Verification items for the finished model (mm, model axes). A direction names the side the tool comes from. Give positions to 0.01 mm unless a question says otherwise; leave off trailing zeros. Use a Markdown table: item, result.
from build123d import *

# Parameters (mm, degrees)
CUT_EXTRUDE_1_DEPTH         = 298.8022876
CUT_EXTRUDE_1_DEPTH_BACK    = 298.8022876
SKETCH_2_W                  = 19
SKETCH_2_H                  = 9.5
SKETCH_3_R                  = 55
EXTRUDE_1_DEPTH             = 1.5125
SKETCH_4_W                  = 19
SKETCH_4_H                  = 9.5
CUT_EXTRUDE_2_DEPTH         = 2
HOLE_WIZARD_M41_D           = 4.5
PATTERN_CIRCULAR_1_COUNT    = 4
HOLE_WIZARD_M42_D           = 4.5
HOLE_WIZARD_M42_CSINK_D     = 4.55
HOLE_WIZARD_M42_CSINK_ANGLE = 90


with BuildPart() as part:
    # Эскиз1 → Повернуть1 (revolve)
    with BuildSketch(Plane(origin=(0, 0, 0), x_dir=(1, 0, 0), z_dir=(0, 1, 0)), mode=Mode.PRIVATE) as revolve_1_sk:
        Polygon((0, 0), (200, 0), (200, -20), (210, -22.05), (210, 10), (0, 10), align=None)
    revolve(revolve_1_sk.sketch.rotate(Axis((0, 0, -10), (0, 0, 1)), 180), axis=Axis((0, 0, -10), (0, 0, 1)))

    # Эскиз2 → Вырез-Вытянуть1 (cut, two sides: drawn at the far end of the back side and taken through both)
    with BuildSketch(Plane.XY.offset(-CUT_EXTRUDE_1_DEPTH_BACK)):
        Rectangle(SKETCH_2_W, SKETCH_2_H)
    extrude(amount=CUT_EXTRUDE_1_DEPTH + CUT_EXTRUDE_1_DEPTH_BACK, mode=Mode.SUBTRACT)

    # Эскиз3 → Бобышка-Вытянуть1 (add)
    with BuildSketch(Plane.XY):
        with Locations(Location((0, 0, 0), (0, 0, 180))):
            Circle(SKETCH_3_R)
    extrude(amount=EXTRUDE_1_DEPTH)

    # Эскиз4 → Вырез-Вытянуть2 (cut)
    with BuildSketch(Plane.XY.offset(1.5125)):
        Rectangle(SKETCH_4_W, SKETCH_4_H)
    extrude(amount=-CUT_EXTRUDE_2_DEPTH, mode=Mode.SUBTRACT)

    # Отверстие с зазором M41 (through all)
    with Locations(Plane(origin=(0, 45, 1.5125), x_dir=(1, 0, 0), z_dir=(0, 0, 1))):
        with Locations((0, 0)):
            hole_wizard_m41 = Hole(HOLE_WIZARD_M41_D / 2)

    # Круговой массив1: Отверстие с зазором M41 ×4 about axis
    pattern_circular_1_axis = Axis((0, 0, 0), (0, 0, 1))
    for i in range(1, PATTERN_CIRCULAR_1_COUNT):
        add(hole_wizard_m41.rotate(pattern_circular_1_axis, i * 360 / PATTERN_CIRCULAR_1_COUNT), mode=Mode.SUBTRACT)

    # Отверстие с зазором M42 (through all)
    with Locations(Plane(origin=(-14.5, 15, -10), x_dir=(-1, 0, 0), z_dir=(0, 0, -1))):
        with Locations((0, 0), (-29, 0), (-29, -30), (0, -30)):
            CounterSinkHole(HOLE_WIZARD_M42_D / 2, HOLE_WIZARD_M42_CSINK_D / 2, counter_sink_angle=HOLE_WIZARD_M42_CSINK_ANGLE)


solid = part.part
(1) Gauge pin test, flat ends, axial feed: P1, Ø8, axis at x = -8, z = 6.5, coming from the +Y side; P2, Ø6, axis at x = 109.5, z = 9.5, coming from the +Y side; P3, Ø10, axis at y = 138.5, z = 14.5, coming from the +X side. Record the tip position at first contact, or that the pin passes through.
Results below:
| item | result |
|---|---|
| P1 | y = 209.96 |
| P2 | y = 180.99 |
| P3 | x = 162.1 |
(2) Set-up check for faces 4 (the flat face through (0, -4.75, -4)), 5 (the flat face through (1, 11, 1.512)): record each of +Z, -Z, +X, -X, +Y, -Y from which the full face is reachable in a straight line by a thin tool's end or side.
Results below:
| item | result |
|---|---|
| face 4 | +Z, -Z |
| face 5 | +Z |
(3) Draft check along X on faces 1 (the cylindrical face through (-200.3, -63.08, 5.8)), 2 (the flat face through (-9.5, 0, -4)), 3 (the flat face through (3, 44, -10)). Enter one of: +X half, -X half, draft (parallel to the pull), parting line (faces both ways), or undercut.
Results below:
| item | result |
|---|---|
| face 1 | parting line |
| face 2 | undercut |
| face 3 | draft |
(4) Material ranges on line 1 (Y direction, x = 0, z = -6); line 2 (X direction, y = -15, z = -6.5); line 3 (Z direction, x = -10, y = -34), recorded low to high.
Results below:
| item | result |
|---|---|
| line 1 | -210 to -47.25, -42.75 to -4.75, 4.75 to 42.75, 47.25 to 210 |
| line 2 | -209.46 to -16.75, -12.25 to 12.25, 16.75 to 209.46 |
| line 3 | -10 to 1.51 |
